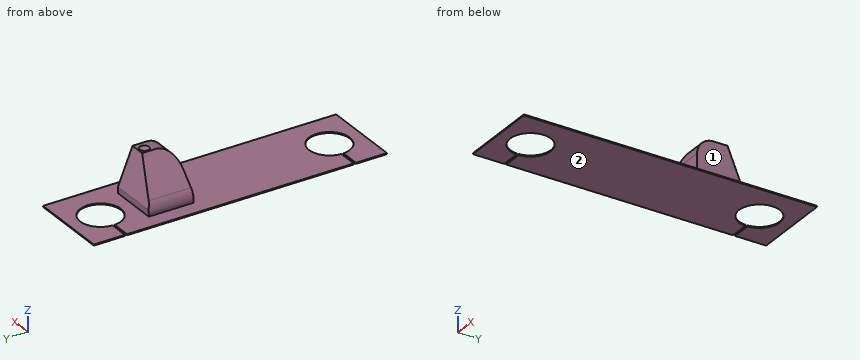
```python
from build123d import *

# Parameters (mm, degrees)
F1_DEPTH     = 0.5
F2_W         = 23.2733339071
F2_H         = 21.7338502407
F3_DEPTH     = 20
F6_R         = 2.3033864012
F5_R         = 2.4232405009
F8_SIZE      = 16
F9_R         = 8
F10_R        = 7
F11_SIZE     = 7
F12_T1_DEPTH = 66.1267417653


# Not quite as in the source:
# - a fillet or chamfer that OpenCascade refuses, or shapes differently, is made with other operations: its cross-section is extruded or revolved along the edge and cut away or added


with BuildPart() as f1:
    # F0 (on Top) → F1 (new body)
    with BuildSketch(Plane.XY):
        with BuildLine():
            Line((19.1950201988, 70.8673447371), (-19.1950201988, 70.8673447371))
            Line((-19.1950201988, 70.8673447371), (-19.1950201988, 55.8184058152))
            Line((-19.1950201988, 55.8184058152), (-9.8077457496, 55.8184058152))
            ThreePointArc((-9.8077457496, 55.8184058152), (9.8204918965, 55.3182214499), (-9.8077457496, 54.8180370845))
            Line((-9.8077457496, 54.8180370845), (-19.1950201988, 54.8180370845))
            Line((-19.1950201988, 54.8180370845), (-19.1950201988, -54.8180370845))
            Line((-19.1950201988, -54.8180370845), (-9.8077457496, -54.8180370845))
            ThreePointArc((-9.8077457496, -54.8180370845), (9.8204918965, -55.3182214499), (-9.8077457496, -55.8184058152))
            Line((-9.8077457496, -55.8184058152), (-19.1950201988, -55.8184058152))
            Line((-19.1950201988, -55.8184058152), (-19.1950201988, -70.8673447371))
            Line((-19.1950201988, -70.8673447371), (19.1950201988, -70.8673447371))
            Line((19.1950201988, -70.8673447371), (19.1950201988, 70.8673447371))
        make_face()
    extrude(amount=F1_DEPTH)

    # F2 (on face) → F3 (join)
    with BuildSketch(Plane.XY.offset(0.5)):
        with Locations((0, 28.6038741469)):
            Rectangle(F2_W, F2_H)
    extrude(amount=F3_DEPTH)

    # F6 (on face) → F7 section 0
    with BuildSketch(Plane.XY.offset(20.5)):
        with Locations((7.3801875114, 29.4457376003)):
            Circle(F6_R)
    # F5 (on offset) → F7 section 1
    with BuildSketch(Plane.XY.offset(0.5)):
        with Locations((-7.0039108396, 29.0047153831)):
            Circle(F5_R)
    loft(mode=Mode.SUBTRACT)

    # F8
    f8_edges = [f1.edges().sort_by_distance(p)[0] for p in [
        (-11.636667, 28.603874, 20.5),
    ]]
    chamfer(f8_edges, length=F8_SIZE)

    # F9
    f9_edges = [f1.edges().sort_by_distance(p)[0] for p in [
        (8, 17.736949, 20.5),
    ]]
    fillet(f9_edges, radius=F9_R)

    # F10
    f10_edges = [f1.edges().sort_by_distance(p)[0] for p in [
        (-11.636667, 28.603874, 4.5),
    ]]
    fillet(f10_edges, radius=F10_R)

    # F11
    f11_edges = [f1.edges().sort_by_distance(p)[0] for p in [
        (8, 39.470799, 20.5),
    ]]
    chamfer(f11_edges, length=F11_SIZE)

    # F12: chamfer of 10 on 1 edges, made by hand

    # F12_s2 → F12_t1 (cut)
    with BuildSketch(Plane.YZ.offset(-28.5633708826)):
        Polygon((39.4707992673, 3.5), (32.3997314554, 20.5710678119), (39.4707992673, 13.5), align=None)
    extrude(amount=F12_T1_DEPTH, mode=Mode.SUBTRACT)


solid = f1.part
```
Work out the finished part from the listing and answer in its coordinate system (mm). Face numbers are marked on the shaded views. A direction names the side the tool comes from. Give positions to 0.01 mm unless a question says otherwise; leave off trailing zeros. Order: outer loops, then holes, each group sorted by start corner. A loop starts at its lowest first (then second) coordinate and runs counter-clockwise, first axis right, second up.
1. Section C-C, the plane y = -36 is taken. Determine the outline of the cut face in (x, z), and give its area (3 significant figures).
Result sheet:
outline: (-19.2, 0) - (19.2, 0) - (19.2, 0.5) - (-19.2, 0.5) - close
area: 19.2 mm2
2. For the marked faces 1 and 2, determine the directions among +Z, -Z, +X, -X, +Y, -Y from which every point of the face is accessible in a straight line to the end or side of a thin tool.
Result sheet:
face 1: +Z, +X, +Y, -Y
face 2: -Z, +X, -X, +Y, -Y
3. Each of these flat-tipped pins is pushed along its axis until it touches: P1, Ø0.6, axis at y = 31.5, z = 1.5, coming from the -X side; P2, Ø0.9, axis at x = -4, z = 2.5, coming from the +Y side; P3, Ø1.5, axis at y = 24.5, z = 7.5, coming from the -X side. Where does it stop, or does it pass through?
Result sheet:
P1: stops at x = -11.64
P2: stops at y = 39.47
P3: stops at x = -9.39
4. Straight lines are drawn through the part: L1, parallel to Y at x = 0, z = 0.15; L2, parallel to Z at x = 12, y = -65; L3, parallel to Y at x = 4, z = 14.25. For each, find the intervals that lie inside material, in ascending order.
Result sheet:
L1: y = -70.87 to -65.14, -45.5 to 45.5, 65.14 to 70.87
L2: z = 0 to 0.5
L3: y = 17.93 to 27.25, 31.37 to 35.02
5. Section A-A, the plane x = -14 is taken. Determine the outline of the cut face in (y, z), and give its area (3 significant figures).
Result sheet:
outline: (-70.87, 0) - (-55.82, 0) - (-55.82, 0.5) - (-70.87, 0.5) - close; (-54.82, 0) - (54.82, 0) - (54.82, 0.5) - (-54.82, 0.5) - close; (55.82, 0) - (70.87, 0) - (70.87, 0.5) - (55.82, 0.5) - close
area: 69.9 mm2
6. Section B-B, the plane x = 0 is taken. Give the number of separate pieces and of enclosed holes in the cut face, and give its area (3 significant figures).
Result sheet:
separate pieces: 3
enclosed holes: 1
area: 333 mm2
